For this review, take the finished solid that the model builds, in its own axes (mm). Face numbers are marked on the shaded views. A direction names the side the tool comes from. Give positions to 0.01 mm unless a question says otherwise; leave off trailing zeros. Order: outer loops, then holes, each group sorted by start corner. A loop starts at its lowest first (then second) coordinate and runs counter-clockwise, first axis right, second up. Notation, with made-up numbers: (67, 44.5) -> (82, 44.5) arc R21 cw to (82, 51.5) -> close; hole circle Ø7 at (84, 52). An arc over 180 degrees is marked (long way). Return JSON: item names as keys, results as strings. Group by question number.
1) Add section D-D (x = -15). Give the boundary of the cut face in (y, z).
2) Insertion check: P1, Ø25, axis at x = 1, y = 11.5, coming from the +Z side; P2, Ø12, axis at y = 8.5, z = -7.5, coming from the -X side; P3, Ø4, axis at x = -5.5, y = -0.5, coming from the -Z side; P4, Ø5, axis at y = 7.5, z = -0.5, coming from the +X side. Each pin has a flat end and moves straight along its axis. Give the tip position at first contact, or say it passes through.
3) Add section C-C (z = -1.5). State how many separate pieces and enclosed holes the cut face has, then the cut area to 3 significant figures.
4) Add section B-B (y = 0). Give the boundary of the cut face in (x, z).
5) Add section A-A (x = 0). Give the boundary of the cut face in (y, z), then the cut area to 3 significant figures.
6) The part is to be moulded in two halves that separate along X. For the marked faces 1, 2 and 3, say which applies: released by +X, released by -X, zero draft, split by the parting line, or undercut.
7) To check wall thickness, follow line 1 along Y through (x, z) = (0, 13.5); line 2 along Y through (x, z) = (0, 4.75); line 3 along Z through (x, y) = (-7.5, 16). State the ranges of each line that lie inside material, in increasing order.
8) For the marked faces 4 and 5, list the 3-axis set-ups (+Z, -Z, +X, -X, +Y, -Y) from which the entire face can be reached by the end or side of a thin tool; tool diameter is ignored.
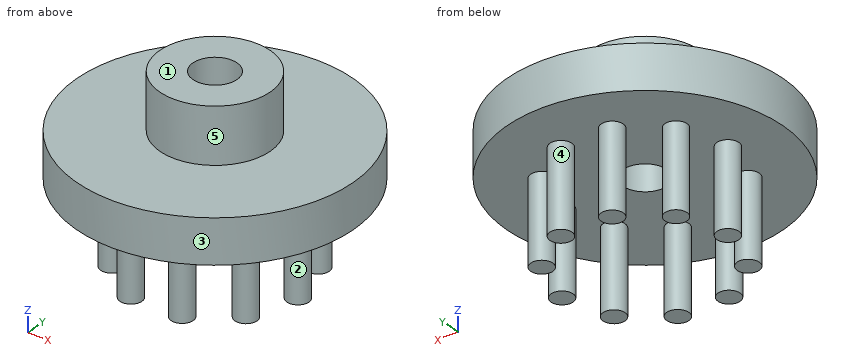
from build123d import *
from build123d.topology import SkipClean

# Parameters (mm, degrees)
SKETCH1_R               = 25
BOSS_EXTRUDE1_DEPTH     = 8
SKETCH2_R               = 2
BOSS_EXTRUDE2_DEPTH     = 15
CUT_EXTRUDE1_DEPTH      = 39.405728739
CUT_EXTRUDE1_DEPTH_BACK = 39.405728739
SKETCH3_R               = 4
SKETCH4_R               = 10
SKETCH4_R_2             = 4
BOSS_EXTRUDE3_DEPTH     = 10


with BuildPart() as part:
    # Sketch1 → Boss-Extrude1 (new body)
    with BuildSketch(Plane.XY):
        Circle(SKETCH1_R)
    extrude(amount=BOSS_EXTRUDE1_DEPTH)

    # Sketch2 → Boss-Extrude2 (add)
    with BuildSketch(Plane(origin=(0, 0, 0), x_dir=(-1, 0, 0), z_dir=(0, 0, -1))):
        with Locations(Location((15, 0, 0), (0, 0, 180))):
            Circle(SKETCH2_R)
        with Locations(Location((12.135254916, -8.816778784, 0), (0, 0, 180))):
            Circle(SKETCH2_R)
        with Locations(Location((4.635254916, -14.265847744, 0), (0, 0, 180))):
            Circle(SKETCH2_R)
        with Locations(Location((-4.635254916, -14.265847744, 0), (0, 0, 180))):
            Circle(SKETCH2_R)
        with Locations(Location((-12.135254916, -8.816778784, 0), (0, 0, 180))):
            Circle(SKETCH2_R)
        with Locations(Location((-15, 0, 0), (0, 0, 180))):
            Circle(SKETCH2_R)
        with Locations(Location((-12.135254916, 8.816778784, 0), (0, 0, 180))):
            Circle(SKETCH2_R)
        with Locations(Location((-4.635254916, 14.265847744, 0), (0, 0, 180))):
            Circle(SKETCH2_R)
        with Locations(Location((4.635254916, 14.265847744, 0), (0, 0, 180))):
            Circle(SKETCH2_R)
        with Locations(Location((12.135254916, 8.816778784, 0), (0, 0, 180))):
            Circle(SKETCH2_R)
    extrude(amount=BOSS_EXTRUDE2_DEPTH)

    # Sketch3 → Cut-Extrude1 (cut, two sides: drawn at the far end of the back side and taken through both)
    with BuildSketch(Plane(origin=(0, 0, 0), x_dir=(-1, 0, 0), z_dir=(0, 0, -1)).offset(-CUT_EXTRUDE1_DEPTH_BACK)):
        Circle(SKETCH3_R)
    extrude(amount=CUT_EXTRUDE1_DEPTH + CUT_EXTRUDE1_DEPTH_BACK, mode=Mode.SUBTRACT)

    # Sketch4 → Boss-Extrude3 (add)
    with SkipClean():  # the faces are left unmerged after this step: merging them gives an invalid solid
        with BuildSketch(Plane.XY.offset(8)):
            Circle(SKETCH4_R)
            Circle(SKETCH4_R_2, mode=Mode.SUBTRACT)
        extrude(amount=BOSS_EXTRUDE3_DEPTH)


solid = part.part
Evaluation:
{
 "1": {"outline": "(-20, 0) -> (-2, 0) -> (-2, -15) -> (2, -15) -> (2, 0) -> (20, 0) -> (20, 8) -> (-20, 8) -> close"},
 "2": {"P1": "z = 18", "P2": "x = -14.14", "P3": "z = 0", "P4": "x = 24.48"},
 "3": {"separate pieces": "10", "enclosed holes": "0", "area": "126 mm^2"},
 "4": {"outline": "(-25, 0) -> (-17, 0) -> (-17, -15) -> (-13, -15) -> (-13, 0) -> (-4, 0) -> (-4, 18) -> (-10, 18) -> (-10, 8) -> (-25, 8) -> close; (4, 0) -> (13, 0) -> (13, -15) -> (17, -15) -> (17, 0) -> (25, 0) -> (25, 8) -> (10, 8) -> (10, 18) -> (4, 18) -> close"},
 "5": {"outline": "(-25, 0) -> (-4, 0) -> (-4, 18) -> (-10, 18) -> (-10, 8) -> (-25, 8) -> close; (4, 0) -> (25, 0) -> (25, 8) -> (10, 8) -> (10, 18) -> (4, 18) -> close", "area": "456 mm^2"},
 "6": {"face 1": "zero draft", "face 2": "undercut", "face 3": "split by the parting line"},
 "7": {"line 1": "-10 to -4, 4 to 10", "line 2": "-25 to -4, 4 to 25", "line 3": "0 to 8"},
 "8": {"face 4": "-Z", "face 5": "+Z"}
}
